Model file for the job. Use its own axes, mm. A direction names the side the tool comes from. Coordinates: 2 decimals unless noted, no trailing zeros. Loops run counter-clockwise (first coordinate to the right, second up) from the corner with the lowest first, then second, coordinate; pieces in that order, holes last.
from build123d import *

# Parameters (mm, degrees)
PAD059_DEPTH            = 5
SKETCH256_R             = 1.525
POCKET023_DEPTH         = 5.001
SKETCH254_R             = 1.65
POCKET024_DEPTH         = 10.062801
SKETCH258_R             = 1.45
POCKET025_DEPTH         = 8
BODY018_PLACEMENT_ANGLE = 90


with BuildPart() as part:
    # Sketch255 → Revolution006 (revolve)
    with BuildSketch(Plane.XZ):
        Polygon((1.65, -18), (1.65, -8), (1.45, -8), (1.45, 0), (5, 0), (5, -18), align=None)
    revolve(axis=Axis((0, 0, 0), (0, 0, 1)))

    # Sketch257 → Pad059 (new body)
    with BuildSketch(Plane.XZ):
        with BuildLine():
            ThreePointArc((-1.255464, -10.137095), (0, -18.061801), (1.255464, -10.137095))
            Line((1.255464, -10.137095), (1.255464, 0))
            Line((1.255464, 0), (-1.255464, 0))
            Line((-1.255464, 0), (-1.255464, -10.137095))
        make_face()
    extrude(amount=PAD059_DEPTH)

    # Sketch256 → Pocket023 (cut, through all)
    with BuildSketch(Plane.XZ):
        with Locations((0, -14.232587)):
            Circle(SKETCH256_R)
    extrude(amount=POCKET023_DEPTH, mode=Mode.SUBTRACT)

    # Sketch254 → Pocket024 (cut, through all)
    with BuildSketch(Plane.XY.offset(-8)):
        Circle(SKETCH254_R)
    extrude(amount=-POCKET024_DEPTH, mode=Mode.SUBTRACT)

    # Sketch258 → Pocket025 (cut)
    with BuildSketch(Plane.XY):
        Circle(SKETCH258_R)
    extrude(amount=-POCKET025_DEPTH, mode=Mode.SUBTRACT)


with BuildPart() as part_1:
    # Body018 placement: moved
    add(part.part.moved(Location((-53, 3, 45))).rotate(Axis((-53, 3, 45), (1, 0, 0)), BODY018_PLACEMENT_ANGLE))


solid = part_1.part
Q1. Drill centre lines: line 1 (Y direction, x = -53, z = 42.35); line 2 (X direction, y = 18.75, z = 45); line 3 (X direction, y = 5, z = 45). Where is each one in solid material? Low to high.
Answers:
line 1: y = 3 to 15.71, 18.76 to 21.06
line 2: x = -58 to -54.65, -51.35 to -48
line 3: x = -58 to -54.45, -51.55 to -48
Q2. Slice it at C-C (z = 42.75). List the corners of the cut face in (x, y) (3 decimals).
Answers:
outline: (-57.465, 3) - (-48.535, 3) - (-48.535, 21) - (-52.294, 21) arc R4.062 ccw to (-53.706, 21) - (-57.465, 21) - close; hole circle Ø3.05 at (-53, 17.233)
Q3. Slice it at A-A (z = 45). List the corners of the cut face in (x, y).
Answers:
outline: (-58, 3) - (-54.45, 3) - (-54.45, 11) - (-54.65, 11) - (-54.65, 21) - (-58, 21) - close; (-51.55, 3) - (-48, 3) - (-48, 21) - (-51.35, 21) - (-51.35, 11) - (-51.55, 11) - close
Q4. Mould opens along Z. For faces 1 (the flat face through (-51.8, 3, 46.2)), 2 (the cylindrical face through (-53.215, 15.961, 46.636)), 3 (the flat face through (-53, 14, 40)), 4 (the cylindrical face through (-53, 12, 50)) say: +Z half, -Z half, draft (parallel to the pull), parting line (faces both ways), or undercut.
Answers:
face 1: draft
face 2: undercut
face 3: -Z half
face 4: parting line
Q5. Slice it at B-B (x = -53). List the corners of the cut face in (y, z).
Answers:
outline: (3, 40) - (15.71, 40) - (15.71, 43.35) - (11, 43.35) - (11, 43.55) - (3, 43.55) - close; (3, 46.45) - (11, 46.45) - (11, 46.65) - (21, 46.65) - (21, 50) - (3, 50) - close; (18.76, 40) - (21.06, 40) - (21.06, 43.35) - (18.76, 43.35) - close
Q6. Slice it at D-D (y = 20). List the corners of the cut face in (x, z), and give its area (3 significant figures).
Answers:
outline: (-55.74, 40) - (-50.26, 40) - (-50.26, 40.82) arc R5 ccw (long way) to (-55.74, 40.82) - close; hole circle Ø3.3 at (-53, 45)
area: 71.4 mm2
Q7. Flat gauge pins, fed straight in: P1, Ø4, axis at x = -55.5, z = 44.5, coming from the +Y side; P2, Ø1, axis at x = -56, y = 12.5, coming from the -Z side; P3, Ø6, axis at x = -50.5, z = 41.5, coming from the +Y side. Where does each tip first touch, or does it go through?
Answers:
P1: stops at y = 21
P2: stops at z = 40.67
P3: stops at y = 21.06
Q8. Which spindle directions (+Z, -Z, +X, -X, +Y, -Y) get a long thin tool onto all of the face, cutting with end or side? Do faces 5 (the cylindrical face through (-53.16, 21.06, 41)), 6 (the cylindrical face through (-52.45, 6.94, 46.34)). Say none if no direction does.
Answers:
face 5: -Z
face 6: +Y, -Y
